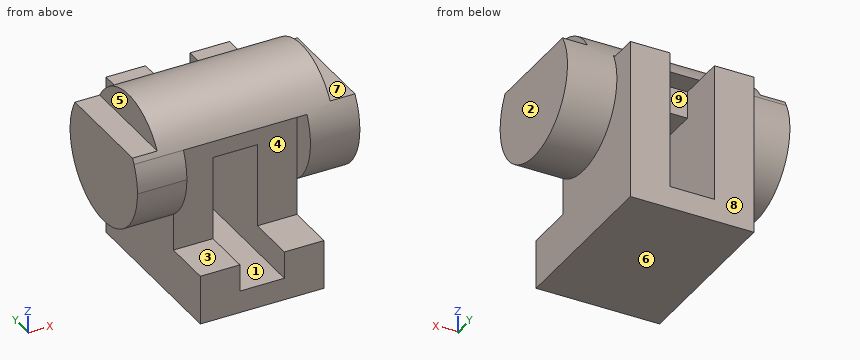
from build123d import *

# Parameters (mm, degrees)
F1_DEPTH  = 70
F2_W      = 16
F2_H      = 50
F3_DEPTH  = 45
F5_DEPTH  = 20
F6_DEPTH  = 90
F10_DEPTH = 10
F12_DEPTH = 10
F13_DEPTH = 20
F16_DEPTH = 50
F17_DEPTH = 25
F18_DEPTH = 5
F19_W     = 18
F19_H     = 19
F20_DEPTH = 50.001
F21_DEPTH = 5
F22_DEPTH = 20


with BuildPart() as f1:
    # F0 (on Front) → F1 (new body)
    with BuildSketch(Plane.XZ):
        Polygon((0, 20), (0, 0), (50, 0), (50, 20), (34, 20), (34, 9), (16, 9), (16, 20), align=None)
    extrude(amount=-F1_DEPTH)

    # F2 (on face) → F3 (join)
    with BuildSketch(Plane.XY.offset(20)):
        with Locations((8, 45)):
            Rectangle(F2_W, F2_H)
        with Locations((42, 45)):
            Rectangle(F2_W, F2_H)
    extrude(amount=F3_DEPTH)

    # F4 (on face) → F5 (join)
    with BuildSketch(Plane(origin=(0, 0, 0), x_dir=(0, -1, 0), z_dir=(-1, 0, 0))):
        with BuildLine():
            ThreePointArc((-20, 35), (-12.639320225, 43.8196601125), (-10, 55))
            ThreePointArc((-10, 55), (-29.8922589078, 79.4726578233), (-57.9128784748, 65))
            Line((-57.9128784748, 65), (-20, 65))
            Line((-20, 65), (-20, 35))
        make_face()
        with BuildLine():
            Line((-20, 65), (-57.9128784748, 65))
            ThreePointArc((-57.9128784748, 65), (-50.5130078141, 35.3952406656), (-20, 35))
            Line((-20, 35), (-20, 65))
        make_face()
    extrude(amount=F5_DEPTH)

    # F6 (add): a face of the model
    f6_faces = [f1.faces().sort_by_distance(p)[0] for p in [
        (-20, 35, 55),
    ]]
    extrude(f6_faces, amount=-F6_DEPTH)

    # F9 (on face) → F10 (cut)
    with BuildSketch(Plane(origin=(-20, 0, 0), x_dir=(0, -1, 0), z_dir=(-1, 0, 0))):
        with BuildLine():
            ThreePointArc((-13.6460271844, 68.0003017268), (-35, 80), (-56.3539728156, 68.0003017268))
            Line((-56.3539728156, 68.0003017268), (-13.6460271844, 68.0003017268))
        make_face()
    extrude(amount=-F10_DEPTH, mode=Mode.SUBTRACT)

    # F11 (on face) → F12 (cut)
    with BuildSketch(Plane.YZ.offset(70)):
        with BuildLine():
            ThreePointArc((56.3539728156, 68.0003017268), (35, 80), (13.6460271844, 68.0003017268))
            Line((13.6460271844, 68.0003017268), (56.3539728156, 68.0003017268))
        make_face()
    extrude(amount=-F12_DEPTH, mode=Mode.SUBTRACT)

    # F8 (on face) → F13 (cut)
    with BuildSketch(Plane(origin=(-20, 0, 0), x_dir=(0, -1, 0), z_dir=(-1, 0, 0))):
        with BuildLine():
            Line((-12.5433961203, 65.9863980535), (-35.1228261001, 65.9863980535))
            Line((-35.1228261001, 65.9863980535), (-35.1228261001, 30.0003017268))
            ThreePointArc((-35.1228261001, 30.0003017268), (-17.3658095239, 37.2789580935), (-10, 55))
            ThreePointArc((-10, 55), (-10.6441475514, 60.6384795383), (-12.5433961203, 65.9863980535))
        make_face()
        with BuildLine():
            Line((-35.1228261001, 30.0003017268), (-35.1228261001, 65.9863980535))
            Line((-35.1228261001, 65.9863980535), (-57.4566038797, 65.9863980535))
            ThreePointArc((-57.4566038797, 65.9863980535), (-56.2416441633, 41.816959636), (-35.1228261001, 30.0003017268))
        make_face()
    extrude(amount=-F13_DEPTH, mode=Mode.SUBTRACT)

    # F15 (on face) + F14 (on face) → F16 (cut)
    with BuildSketch(Plane(origin=(0, 0, 0), x_dir=(0, -1, 0), z_dir=(-1, 0, 0))):
        with BuildLine():
            Line((-70, 65), (-70, 35))
            Line((-70, 35), (-20, 35))
            Line((-20, 35), (-20, 65.9863980535))
            Line((-20, 65.9863980535), (-57.4566038797, 65.9863980535))
            ThreePointArc((-57.4566038797, 65.9863980535), (-57.6901019733, 65.4956787508), (-57.9128784748, 65))
            Line((-57.9128784748, 65), (-70, 65))
        make_face()
    with BuildSketch(Plane(origin=(0, 0, 0), x_dir=(0, -1, 0), z_dir=(-1, 0, 0))):
        with BuildLine():
            Line((-20, 65.9863980535), (-20, 35))
            ThreePointArc((-20, 35), (-12.639320225, 43.8196601125), (-10, 55))
            ThreePointArc((-10, 55), (-10.6441475514, 60.6384795383), (-12.5433961203, 65.9863980535))
            Line((-12.5433961203, 65.9863980535), (-20, 65.9863980535))
        make_face()
    extrude(amount=-F16_DEPTH, mode=Mode.SUBTRACT)

    # F17 (add): a face of the model
    f17_faces = [f1.faces().sort_by_distance(p)[0] for p in [
        (25, 42.476635514, 35),
    ]]
    extrude(f17_faces, amount=F17_DEPTH)

    # F18 (add): a face of the model
    f18_faces = [f1.faces().sort_by_distance(p)[0] for p in [
        (25, 42.476635514, 60),
    ]]
    extrude(f18_faces, amount=F18_DEPTH)

    # F19 (on face) → F20 (cut, through all)
    with BuildSketch(Plane.XZ.offset(-20)):
        with Locations((25, 44.5)):
            Rectangle(F19_W, F19_H)
    extrude(amount=-F20_DEPTH, mode=Mode.SUBTRACT)

    # F21 (cut, through all): a face of the model
    f21_faces = [f1.faces().sort_by_distance(p)[0] for p in [
        (25, 35, 35),
    ]]
    extrude(f21_faces, amount=-F21_DEPTH, mode=Mode.SUBTRACT)

    # F7 (on face) → F22 (join)
    with BuildSketch(Plane(origin=(-20, 0, 0), x_dir=(0, -1, 0), z_dir=(-1, 0, 0))):
        with BuildLine():
            Line((-12.5433961203, 65.9863980535), (-57.4566038797, 65.9863980535))
            ThreePointArc((-57.4566038797, 65.9863980535), (-40.6384795383, 30.6441475514), (-10, 55))
            ThreePointArc((-10, 55), (-10.6441475514, 60.6384795383), (-12.5433961203, 65.9863980535))
        make_face()
    extrude(amount=-F22_DEPTH)


solid = f1.part
Geometry check sheet. Reference: the model listing, model coordinates, mm. Face numbers are marked on the shaded views. A direction names the side the tool comes from. Coordinates: 2 decimals unless noted, no trailing zeros. Loops run counter-clockwise (first coordinate to the right, second up) from the corner with the lowest first, then second, coordinate; pieces in that order, holes last. Notation, with made-up numbers: (13, 47) - (30, 47) arc R28 ccw to (30, 72) - close; hole circle Ø11 at (38, 6). An arc over 180 degrees is marked (long way). Use one line per item in the form item = value. Start each with the question number.
Item 1: Thickness scan on probe 1 along X at (y, z) = (47, 34.5); probe 2 along X at (y, z) = (30, 10); probe 3 along Z at (x, y) = (22.5, 29). Record the ranges inside material, lowest first.
Item 2: Tool access check on the marked faces 1, 2, 3, 4 and 5. Record the directions out of +Z, -Z, +X, -X, +Y, -Y that give a thin tool (end or side, any length) a straight path to the whole face; none if there is none.
Item 3: Section check B-B, the plane x = 45.5. Enter the section's corners in (y, z), and give its area (3 significant figures).
Item 4: Section check A-A, the plane y = 15. Enter the section's corners in (x, z), and give its area (3 significant figures).
Item 5: Section check D-D, the plane z = 41.5. Enter the section's corners in (x, y).
Item 6: Mould release check, pull along Z, two halves, no side actions. Record for the marked faces 6, 7, 8 and 9: +Z half, -Z half, draft (parallel to the pull), parting line (faces both ways), or undercut.
Item 7: Gauge pin test, flat ends, axial feed: pin 1 (5 mm diameter, centred on x = -13, y = 36, fed in from +Z); pin 2 (9 mm diameter, centred on x = 26.5, z = 61, fed in from +Y); pin 3 (4 mm diameter, centred on y = 22.5, z = 26.5, fed in from -X); pin 4 (5.5 mm diameter, centred on x = 24, y = 33.5, fed in from -Z). Record the tip position at first contact, or that the pin passes through.
Item 8: Section check C-C, the plane y = 35. Enter the section's corners in (x, z), and give its area (3 significant figures).
Computed:
q1.probe_1 = -20 to 16, 34 to 70
q1.probe_2 = 0 to 16, 34 to 50
q1.probe_3 = 0 to 9, 54 to 65, 65.99 to 79.27
q2.face_1 = +Y, -Y
q2.face_2 = +Z, -Z, +X, +Y, -Y
q2.face_3 = +X, -X, -Y
q2.face_4 = -Y
q2.face_5 = +Z, -X, +Y, -Y
q3.outline = (0, 0) - (70, 0) - (70, 65) - (20, 65) - (20, 20) - (0, 20) - close; (12.54, 65.99) - (57.46, 65.99) arc R25 ccw to start
q3.area = 4,100 mm2
q4.outline = (-20, 40) - (0, 40) - (0, 65.99) - (50, 65.99) - (50, 40) - (70, 40) - (70, 68) - (60, 68) - (60, 70) - (-10, 70) - (-10, 68) - (-20, 68) - close; (0, 0) - (50, 0) - (50, 20) - (34, 20) - (34, 9) - (16, 9) - (16, 20) - (0, 20) - close
q4.area = 2,160 mm2
q5.outline = (-20, 13.96) - (0, 13.96) - (0, 20) - (16, 20) - (16, 70) - (0, 70) - (0, 56.04) - (-20, 56.04) - close; (34, 20) - (50, 20) - (50, 13.96) - (70, 13.96) - (70, 56.04) - (50, 56.04) - (50, 70) - (34, 70) - close
q6.face_6 = -Z half
q6.face_7 = +Z half
q6.face_8 = draft
q6.face_9 = undercut
q7.pin_1 = 68
q7.pin_2 = 50
q7.pin_3 = 0
q7.pin_4 = 0
q8.outline = (-20, 30) - (0, 30) - (0, 0) - (50, 0) - (50, 30) - (70, 30) - (70, 68) - (60, 68) - (60, 80) - (-10, 80) - (-10, 68) - (-20, 68) - close; hole (0, 65) - (50, 65) - (50, 65.99) - (0, 65.99) - close; hole (16, 9) - (34, 9) - (34, 54) - (16, 54) - close
q8.area = 4,900 mm2
